Work out the finished part from the listing and answer in its coordinate system (mm). Give positions to 0.01 mm unless a question says otherwise; leave off trailing zeros. Loops run counter-clockwise (first coordinate to the right, second up) from the corner with the lowest first, then second, coordinate; pieces in that order, holes last. Notation, with made-up numbers: (-0.75, 3) - (38.25, 3) arc R23 cw to (38.25, 21) - close; hole circle Ø9 at (22, 11.25). An arc over 180 degrees is marked (long way). One line per question, with ' | ' between items.
from build123d import *

# Parameters (mm, degrees)
BOSS_EXTRUDE1_DEPTH = 5
SKETCH5_W           = 5
SKETCH5_H           = 6
BOSS_EXTRUDE7_DEPTH = 32
SKETCH4_R           = 1.4
BOSS_EXTRUDE4_DEPTH = 8


with BuildPart() as part:
    # Sketch1 → Boss-Extrude1 (new body)
    with BuildSketch(Plane.XY):
        Polygon((0, 6.7), (0, 8.05), (5.5, 8.05), (14.2, 8.05), (14.2, -18.95), (146.5, -18.95), (146.5, -42.1), (151.5, -42.1), (151.5, -13.95), (19.2, -13.95), (19.2, 12.9), (5.5, 12.9), (-5, 12.9), (-5, 0), (0, 0), align=None)
    extrude(amount=BOSS_EXTRUDE1_DEPTH)

    # Sketch5 → Boss-Extrude7 (add)
    with BuildSketch(Plane(origin=(0, 0, 0), x_dir=(-1, 0, 0), z_dir=(0, 0, -1))):
        with Locations((-149, -39.1)):
            Rectangle(SKETCH5_W, SKETCH5_H)
    extrude(amount=BOSS_EXTRUDE7_DEPTH)

    # Sketch4 → Boss-Extrude4 (add)
    with BuildSketch(Plane.ZY.offset(-146.5)):
        with Locations(Location((-29, -39.1, 0), (0, 0, 180))):
            Circle(SKETCH4_R)
        with Locations(Location((2, -39.1, 0), (0, 0, 180))):
            Circle(SKETCH4_R)
    extrude(amount=BOSS_EXTRUDE4_DEPTH)


solid = part.part
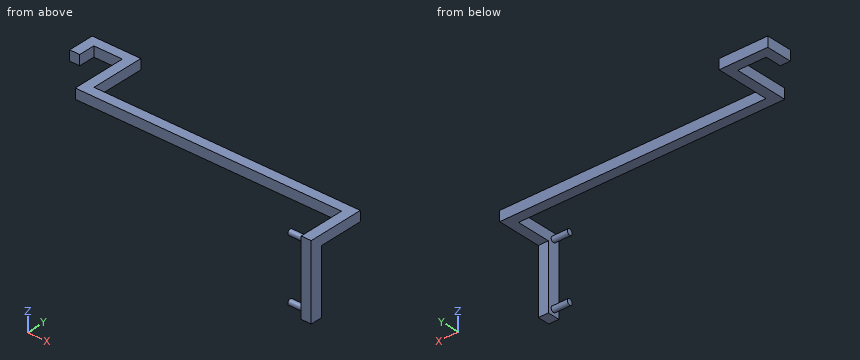
1. Consider L1, parallel to Y at x = 28, z = 1.5; L2, parallel to Z at x = 72, y = -15; L3, parallel to X at y = -39, z = -25.5. Determine where each line is inside the solid, lowest interval first.
Evaluation:
L1: -18.95 to -13.95 | L2: 0 to 5 | L3: 146.5 to 151.5
2. Flat-ended cylindrical pins translate along their axes: pin 1 (5.5 mm diameter, centred on y = -4.5, z = 2.5, fed in from -X); pin 2 (1.4 mm diameter, centred on y = -38.5, z = -29.5, fed in from -X); pin 3 (8 mm diameter, centred on x = 104.5, y = -23.5, fed in from -Z); pin 4 (4 mm diameter, centred on x = 7, z = 3, fed in from -Y). Find the tip coordinate at first contact, or state that the pin passes through.
Evaluation:
pin 1: x = 14.2 | pin 2: x = 138.5 | pin 3: through | pin 4: y = 8.05
3. Find section D-D on z = 2. Write down the section's boundary in (x, y).
Evaluation:
outline: (-5, 0) - (0, 0) - (0, 8.05) - (14.2, 8.05) - (14.2, -18.95) - (146.5, -18.95) - (146.5, -37.7) - (138.5, -37.7) - (138.5, -40.5) - (146.5, -40.5) - (146.5, -42.1) - (151.5, -42.1) - (151.5, -13.95) - (19.2, -13.95) - (19.2, 12.9) - (-5, 12.9) - close
4. Find section A-A on z = -29. Write down the section's boundary in (x, y), then the cut area to 3 significant figures.
Evaluation:
outline: (138.5, -40.5) - (146.5, -40.5) - (146.5, -42.1) - (151.5, -42.1) - (151.5, -36.1) - (146.5, -36.1) - (146.5, -37.7) - (138.5, -37.7) - close | area: 52.4 mm2
5. Find section B-B on y = -39.1. Write down the section's boundary in (x, z), then the cut area to 3 significant figures.
Evaluation:
outline: (138.5, -30.4) - (146.5, -30.4) - (146.5, -32) - (151.5, -32) - (151.5, 5) - (146.5, 5) - (146.5, 3.4) - (138.5, 3.4) - (138.5, 0.6) - (146.5, 0.6) - (146.5, -27.6) - (138.5, -27.6) - close | area: 230 mm2
6. Find section C-C on x = 61. Write down the section's boundary in (y, z), then the cut area to 3 significant figures.
Evaluation:
outline: (-18.95, 0) - (-13.95, 0) - (-13.95, 5) - (-18.95, 5) - close | area: 25.0 mm2
